Drawing for the job (mm, zero at the part's lowest x, y, z). A direction names the side the tool comes from. Give positions to 0.01 mm unless a question says otherwise; leave off trailing zeros. Order: outer loops, then holes, each group sorted by start corner. A loop starts at its lowest first (then second) coordinate and runs counter-clockwise, first axis right, second up. Notation, with made-up numbers: (39.5, 47) - (71.5, 47) arc R29 cw to (71.5, 69) - close; hole circle Ø5 at (35, 60). An arc over 180 degrees is marked (long way). One line per item, written item: value.
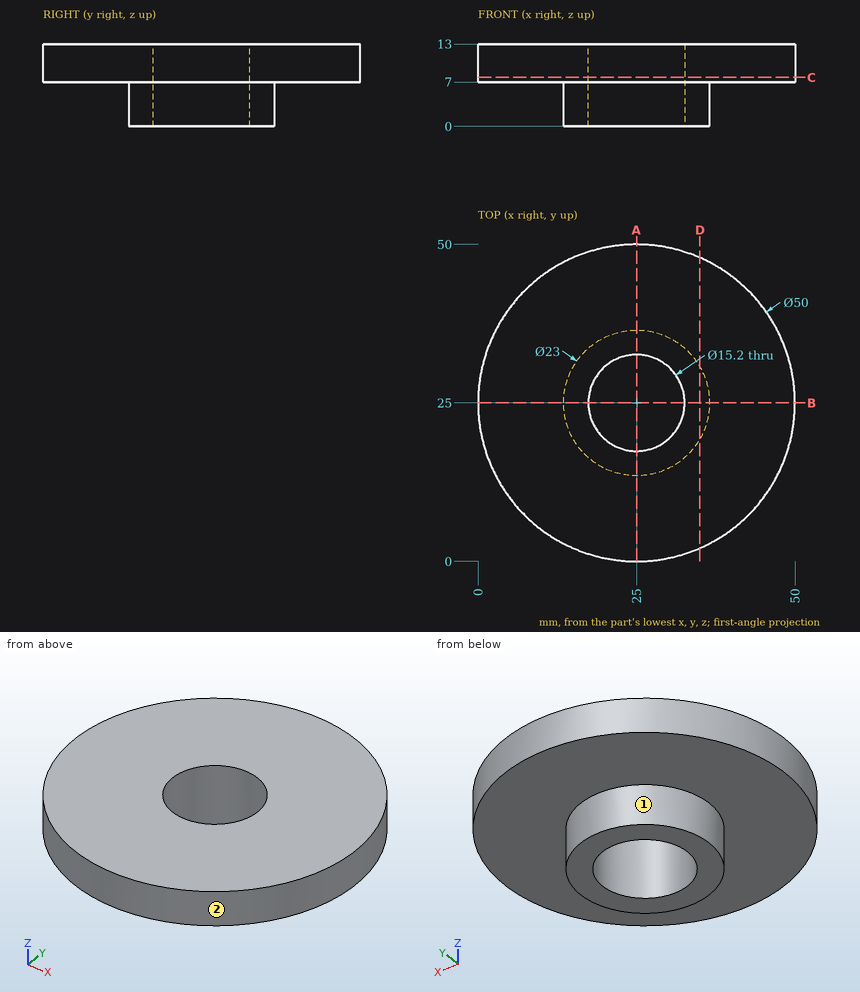
(1) Pin check, flat tips, straight feed: P1, Ø5, axis at x = 24.5, z = 6.5, coming from the -Y side; P2, Ø6, axis at x = 23, y = 43, coming from the -Z side; P3, Ø5, axis at x = 16.5, z = 9, coming from the -Y side. Stop position of each tip, or through.
Completed:
P1: y = 0
P2: z = 7
P3: y = 0.73
(2) Drill centre lines: line 1 (Y direction, x = 25, z = 4.25); line 2 (Z direction, x = 47.5, y = 17); line 3 (Y direction, x = 26, z = 6.5). Where is each one in solid material? Low to high.
Completed:
line 1: 13.5 to 17.4, 32.6 to 36.5
line 2: 7 to 13
line 3: 13.54 to 17.47, 32.53 to 36.46
(3) Slice it at C-C, the plane z = 7.75. Give the cut face in (x, y).
Completed:
outline: circle Ø50 at (25, 25); hole circle Ø15.2 at (25, 25)
(4) 3-axis set-ups, long thin cutter, end or side, ignore diameter. For the marked faces 1 and 2: which of +Z, -Z, +X, -X, +Y, -Y reach the whole face in a straight line?
Completed:
face 1: -Z
face 2: +Z, -Z
(5) Slice it at D-D, the plane x = 35. Give the cut face in (y, z), and give its area (3 significant figures).
Completed:
outline: (2.09, 7) - (19.32, 7) - (19.32, 0) - (30.68, 0) - (30.68, 7) - (47.91, 7) - (47.91, 13) - (2.09, 13) - close
area: 354 mm²
(6) Slice it at A-A, the plane x = 25. Give the cut face in (y, z), and give its area (3 significant figures).
Completed:
outline: (0, 7) - (13.5, 7) - (13.5, 0) - (17.4, 0) - (17.4, 13) - (0, 13) - close; (32.6, 0) - (36.5, 0) - (36.5, 7) - (50, 7) - (50, 13) - (32.6, 13) - close
area: 263 mm²
